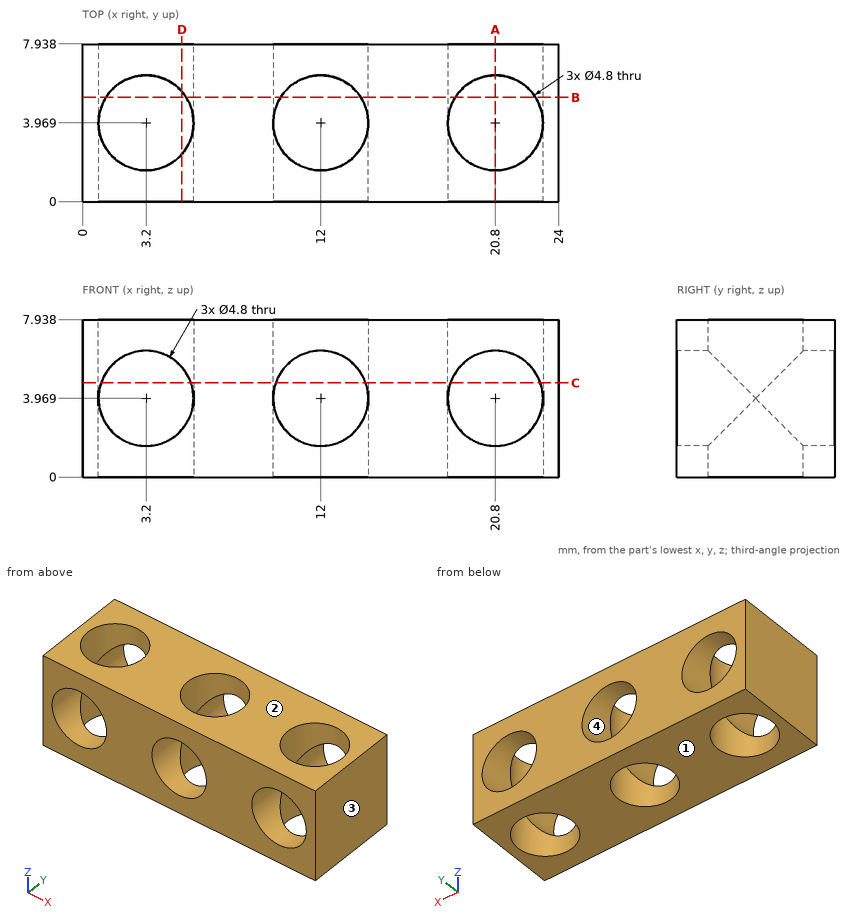
Here's the drawing with two shaded views (mm, measured from the low corner). I have some questions. Round coordinates to 2 decimals unless told otherwise and drop trailing zeros. Write each loop counter-clockwise with the first axis right and the second up, starting at its lowest first coordinate (ties: lowest second). Pieces come first, ordered by that corner, then holes.
(1) If I drill on probe 1 along X at (y, z) = (1.25, 5.25); probe 2 along X at (y, z) = (5, 2.5); probe 3 along Y at (x, z) = (12, 0.9), over which ranges is the centre line in solid material (lowest first)?
Findings below:
probe 1: x = 0 to 1.17, 5.23 to 9.97, 14.03 to 18.77, 22.83 to 24
probe 2: x = 0 to 1.03, 5.37 to 9.83, 14.17 to 18.63, 22.97 to 24
probe 3: y = 0 to 1.57, 6.37 to 7.94
(2) Suppose I cut it at C-C on z = 4.75. Write out the boundary of the cut face in (x, y).
Findings below:
outline: (0, 0) - (0.93, 0) - (0.93, 3.19) arc R2.4 cw to (0.93, 4.75) - (0.93, 7.94) - (0, 7.94) - close; (5.47, 0) - (9.73, 0) - (9.73, 3.19) arc R2.4 cw to (9.73, 4.75) - (9.73, 7.94) - (5.47, 7.94) - (5.47, 4.75) arc R2.4 cw to (5.47, 3.19) - close; (14.27, 0) - (18.53, 0) - (18.53, 3.19) arc R2.4 cw to (18.53, 4.75) - (18.53, 7.94) - (14.27, 7.94) - (14.27, 4.75) arc R2.4 cw to (14.27, 3.19) - close; (23.07, 0) - (24, 0) - (24, 7.94) - (23.07, 7.94) - (23.07, 4.75) arc R2.4 cw to (23.07, 3.19) - close
(3) For pin 1 (4 mm diameter, centred on x = 17.5, z = 2.5, fed in from -Y); pin 2 (3 mm diameter, centred on x = 12, z = 3.97, fed in from +Y), each with a flat end and sliding along its axis, tell me the tip position at first contact or that it passes through.
Findings below:
pin 1: stops at y = 0
pin 2: passes through
(4) Suppose I cut it at A-A on x = 20.8. Write out the boundary of the cut face in (y, z).
Findings below:
outline: (0, 0) - (1.57, 0) - (1.57, 1.57) - (0, 1.57) - close; (0, 6.37) - (1.57, 6.37) - (1.57, 7.94) - (0, 7.94) - close; (6.37, 0) - (7.94, 0) - (7.94, 1.57) - (6.37, 1.57) - close; (6.37, 6.37) - (7.94, 6.37) - (7.94, 7.94) - (6.37, 7.94) - close
(5) Thinking about a two-plate mould opening in Z: for the marked faces 1, 2, 3 and 4, which applies, +Z half, -Z half, draft (parallel to the pull), parting line (faces both ways), or undercut?
Findings below:
face 1: -Z half
face 2: +Z half
face 3: draft
face 4: undercut
(6) Suppose I cut it at B-B on y = 5.25. Write out the boundary of the cut face in (x, z).
Findings below:
outline: (0, 0) - (1.17, 0) - (1.17, 2.69) arc R2.4 cw to (1.17, 5.25) - (1.17, 7.94) - (0, 7.94) - close; (5.23, 0) - (9.97, 0) - (9.97, 2.69) arc R2.4 cw to (9.97, 5.25) - (9.97, 7.94) - (5.23, 7.94) - (5.23, 5.25) arc R2.4 cw to (5.23, 2.69) - close; (14.03, 0) - (18.77, 0) - (18.77, 2.69) arc R2.4 cw to (18.77, 5.25) - (18.77, 7.94) - (14.03, 7.94) - (14.03, 5.25) arc R2.4 cw to (14.03, 2.69) - close; (22.83, 0) - (24, 0) - (24, 7.94) - (22.83, 7.94) - (22.83, 5.25) arc R2.4 cw to (22.83, 2.69) - close
(7) Suppose I cut it at D-D on x = 5. Write out the boundary of the cut face in (y, z).
Findings below:
outline: (0, 0) - (2.38, 0) - (2.38, 2.38) - (0, 2.38) - close; (0, 5.56) - (2.38, 5.56) - (2.38, 7.94) - (0, 7.94) - close; (5.56, 0) - (7.94, 0) - (7.94, 2.38) - (5.56, 2.38) - close; (5.56, 5.56) - (7.94, 5.56) - (7.94, 7.94) - (5.56, 7.94) - close
